```python
from build123d import *

# Parameters (mm, degrees)
CROQUIS1_R              = 1.392405063
CROQUIS1_R_2            = 1.113924051
SALIENTE_EXTRUIR1_DEPTH = 3
CROQUIS8_R              = 1.18
CORTAR_EXTRUIR1_DEPTH   = 10


with BuildPart() as part:
    # Croquis1 → Saliente-Extruir1 (new body)
    with BuildSketch(Plane.XY):
        with BuildLine():
            Line((73.906046363, 79.342028473), (73.906046363, 31.801341312))
            ThreePointArc((73.906046363, 31.801341312), (72.740829217, 28.988258277), (69.927746182, 27.823041131))
            Line((69.927746182, 27.823041131), (49.927651758, 27.823041131))
            ThreePointArc((49.927651758, 27.823041131), (48.521110241, 28.405649704), (47.938501668, 29.812191222))
            Line((47.938501668, 29.812191222), (41.473763874, 29.812191222))
            Line((41.473763874, 29.812191222), (41.473763874, 25.833891041))
            ThreePointArc((41.473763874, 25.833891041), (40.017242442, 22.317537246), (36.500888648, 20.861015815))
            Line((36.500888648, 20.861015815), (-3.002012677, 20.861015815))
            ThreePointArc((-3.002012677, 20.861015815), (-5.463460333, 21.880580817), (-6.483025335, 24.342028473))
            ThreePointArc((-6.483025335, 24.342028473), (-7.502590337, 26.803476129), (-9.964037993, 27.823041131))
            Line((-9.964037993, 27.823041131), (-31.953282507, 27.823041131))
            ThreePointArc((-31.953282507, 27.823041131), (-34.697951359, 28.916679938), (-35.931582688, 31.601341312))
            Line((-35.931582688, 31.601341312), (-35.931582688, 79.142028473))
            ThreePointArc((-35.931582688, 79.142028473), (-34.912017686, 81.603476129), (-32.45057003, 82.623041131))
            Line((-32.45057003, 82.623041131), (-24.991257191, 82.623041131))
            Line((-24.991257191, 82.623041131), (-24.991257191, 87.098628835))
            ThreePointArc((-24.991257191, 87.098628835), (-23.971692189, 89.560076491), (-21.510244533, 90.579641493))
            Line((-21.510244533, 90.579641493), (-9.964037993, 90.579641493))
            ThreePointArc((-9.964037993, 90.579641493), (-7.502590337, 91.599206495), (-6.483025335, 94.060654151))
            ThreePointArc((-6.483025335, 94.060654151), (-5.463460333, 96.522101807), (-3.002012677, 97.541666809))
            Line((-3.002012677, 97.541666809), (36.500888648, 97.541666809))
            ThreePointArc((36.500888648, 97.541666809), (40.017242442, 96.085145378), (41.473763874, 92.568791583))
            Line((41.473763874, 92.568791583), (41.473763874, 88.590491402))
            Line((41.473763874, 88.590491402), (47.938501668, 88.590491402))
            ThreePointArc((47.938501668, 88.590491402), (48.521110241, 89.99703292), (49.927651758, 90.579641493))
            Line((49.927651758, 90.579641493), (59.484708207, 90.579641493))
            ThreePointArc((59.484708207, 90.579641493), (61.946155863, 89.560076491), (62.965720865, 87.098628835))
            Line((62.965720865, 87.098628835), (62.965720865, 82.823041131))
            Line((62.965720865, 82.823041131), (70.425033704, 82.823041131))
            ThreePointArc((70.425033704, 82.823041131), (72.886481361, 81.803476129), (73.906046363, 79.342028473))
        make_face()
        with Locations((-28.70264158, 46.569695742)):
            Circle(CROQUIS1_R, mode=Mode.SUBTRACT)
        with Locations((-28.70264158, 71.632986882)):
            Circle(CROQUIS1_R, mode=Mode.SUBTRACT)
        with Locations((66.677105255, 46.569695742)):
            Circle(CROQUIS1_R, mode=Mode.SUBTRACT)
        with Locations((66.677105255, 71.632986882)):
            Circle(CROQUIS1_R, mode=Mode.SUBTRACT)
        with Locations((6.455586268, 91.17638652)):
            Circle(CROQUIS1_R, mode=Mode.SUBTRACT)
        with Locations((31.518877407, 91.17638652)):
            Circle(CROQUIS1_R, mode=Mode.SUBTRACT)
        with Locations((6.455586268, 27.026296104)):
            Circle(CROQUIS1_R, mode=Mode.SUBTRACT)
        with Locations((31.518877407, 27.026296104)):
            Circle(CROQUIS1_R, mode=Mode.SUBTRACT)
        with Locations((0.125454864, 83.46842992)):
            Circle(CROQUIS1_R_2, mode=Mode.SUBTRACT)
        with Locations((0.125454864, 34.734252705)):
            Circle(CROQUIS1_R_2, mode=Mode.SUBTRACT)
        with Locations((57.810807486, 34.734252705)):
            Circle(CROQUIS1_R_2, mode=Mode.SUBTRACT)
        with Locations((57.810807486, 83.46842992)):
            Circle(CROQUIS1_R_2, mode=Mode.SUBTRACT)
    extrude(amount=SALIENTE_EXTRUIR1_DEPTH)

    # Croquis8 → Cortar-Extruir1 (cut)
    with BuildSketch(Plane.XY.offset(3)):
        with Locations((0.125454864, 34.734252705)):
            Circle(CROQUIS8_R)
        with Locations((57.810807486, 34.734252705)):
            Circle(CROQUIS8_R)
        with Locations((0.125454864, 83.46842992)):
            Circle(CROQUIS8_R)
        with Locations((57.810807486, 83.46842992)):
            Circle(CROQUIS8_R)
    extrude(amount=-CORTAR_EXTRUIR1_DEPTH, mode=Mode.SUBTRACT)


solid = part.part
```
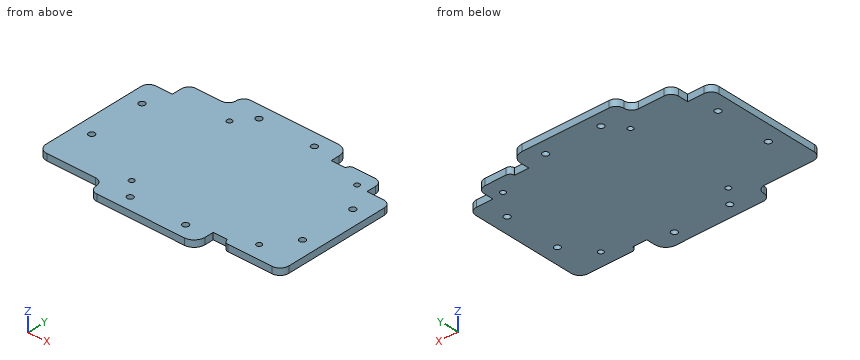
Could you check a few things on this model? Use its own coordinates, in mm. Give positions to 0.01 mm unless a question says otherwise; leave off trailing zeros. Write each loop counter-clockwise with the first axis right and the second up, starting at its lowest first coordinate (ties: lowest second). Pieces come first, ordered by that corner, then holes. Notation, with made-up numbers: (-24.75, 0.25) -> (26.25, 0.25) arc R25 ccw to (26.25, 38.25) -> close; hole circle Ø6 at (19.25, -40). An arc over 180 degrees is marked (long way). Write each question's results on one line, items separated by ' | '.
1. Will these pins go through, and if not, where does the flat tip stop? pin 1 Ø0.9 at (y, z) = (86, 1) entering from +X; pin 2 Ø1 at (x, z) = (52, 2) entering from +Y; pin 3 Ø0.9 at (x, z) = (46, 1) entering from -Y.
Check sheet entries:
pin 1: stops at x = 62.97 | pin 2: stops at y = 90.58 | pin 3: stops at y = 29.81
2. I want a section at B-B, the plane x = 43. Write out the boundary of the cut face in (y, z), then the cut area to 3 significant figures.
Check sheet entries:
outline: (29.81, 0) -> (88.59, 0) -> (88.59, 3) -> (29.81, 3) -> close | area: 176 mm²
3. I want a section at A-A, the plane y = 86. Write out the boundary of the cut face in (x, z).
Check sheet entries:
outline: (-24.99, 0) -> (62.97, 0) -> (62.97, 3) -> (-24.99, 3) -> close
4. I want a section at C-C, the plane z = 0.55. Count the separate pieces of the cut face and the enclosed holes in it, then the cut area to 3 significant figures.
Check sheet entries:
separate pieces: 1 | enclosed holes: 12 | area: 7,270 mm²
5. I need wall thicknesses on L1, parallel to X at y = 91, z = 2.2; L2, parallel to X at y = 84.5, z = 2.45; L3, parallel to X at y = 85, z = 0.6. Which ranges of each line are inside material? Lowest first, please.
Check sheet entries:
L1: x = -8.31 to 5.07, 7.84 to 30.14, 32.9 to 41.47 | L2: x = -24.99 to -0.45, 0.7 to 57.24, 58.38 to 62.97 | L3: x = -24.99 to 62.97
